The listing builds one solid part. Answer for the finished solid, in the listing's coordinates (mm). Face numbers are marked on the shaded views. Coordinates: 2 decimals unless noted, no trailing zeros. Order: outer loops, then holes, each group sorted by start corner. A loop starts at its lowest first (then second) coordinate and runs counter-clockwise, first axis right, second up. Notation, with made-up numbers: M 52.25,18 L 95.25,18 A22 cw 95.25,29 Z; hole C -34.75,20 d9. An arc over 180 degrees is marked long. One line per item, written item: value. Start each with the question number.
Q1. Determine the mould class of the marked faces 1, 2 and 3 for opening direction X: pulls with the +X half, pulls with the -X half, needs draft (parallel to the pull), parting line crosses it, or undercut.
Q2. The part is cut by section C-C on y = -162. Give the vertices of the cut face in (x, z) (3 decimals).
Q3. Each of these flat-tipped pins is pushed along its axis until it touches: pin 1 Ø11.5 at (x, y) = (-90.4, -156.19) entering from -Z; pin 2 Ø1.5 at (x, z) = (-77.5, 0.5) entering from -Y. Where does it stop, or does it pass through?
Q4. Straight lines are drawn through the part: line 1 along X through (y, z) = (-133.5, 0.65); line 2 along Y through (x, z) = (-100.5, 1.05); line 3 along Y through (x, z) = (-87, 0.25). For each, find the intervals that lie inside material, in ascending order. Write a range as [from, to].
Q5. The part is cut by section A-A on x = -89. Give the vertices of the cut face in (y, z) (3 decimals), then the cut area to 3 significant figures.
Q6. The part is cut by section B-B on z = 2.6. Give the number of separate pieces and of enclosed holes in the cut face, then the cut area to 3 significant figures.
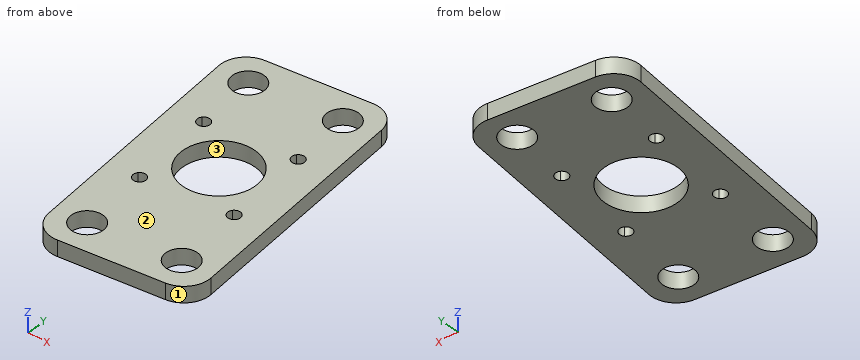
```python
from build123d import *

# Parameters (mm, degrees)
SKETCH1_R           = 7.317167392
SKETCH1_R_2         = 3.175
BOSS_EXTRUDE2_DEPTH = 3.175


with BuildPart() as part:
    # Sketch1 → Boss-Extrude2 (new body)
    with BuildSketch(Plane.XY):
        with BuildLine():
            ThreePointArc((-108.18478159, -135.764097779), (-107.141377815, -132.018654189), (-103.75515137, -130.108023512))
            Line((-103.75515137, -130.108023512), (-83.685324569, -127.667488038))
            ThreePointArc((-83.685324569, -127.667488038), (-79.939880979, -128.710891812), (-78.029250302, -132.097118258))
            Line((-78.029250302, -132.097118258), (-72.356946589, -178.743501511))
            ThreePointArc((-72.356946589, -178.743501511), (-73.400350364, -182.488945101), (-76.78657681, -184.399575778))
            Line((-76.78657681, -184.399575778), (-96.85640361, -186.840111252))
            ThreePointArc((-96.85640361, -186.840111252), (-100.6018472, -185.796707477), (-102.512477877, -182.410481032))
            Line((-102.512477877, -182.410481032), (-108.18478159, -135.764097779))
        make_face()
        with Locations((-90.400440681, -156.188222118)):
            Circle(SKETCH1_R, mode=Mode.SUBTRACT)
        with Locations((-96.362218078, -180.383240442)):
            Circle(SKETCH1_R_2, mode=Mode.SUBTRACT)
        with Locations((-78.813817399, -178.249315979)):
            Circle(SKETCH1_R_2, mode=Mode.SUBTRACT)
        with Locations((-84.179510101, -134.124358848)):
            Circle(SKETCH1_R_2, mode=Mode.SUBTRACT)
        with Locations((-101.72791078, -136.258283311)):
            Circle(SKETCH1_R_2, mode=Mode.SUBTRACT)
        with BuildLine():
            ThreePointArc((-99.257486995, -149.251707821), (-99.470879442, -147.496867753), (-101.225719509, -147.710260199))
            ThreePointArc((-101.225719509, -147.710260199), (-101.012327063, -149.465100267), (-99.257486995, -149.251707821))
        make_face(mode=Mode.SUBTRACT)
        with BuildLine():
            ThreePointArc((-83.677318831, -145.576335736), (-83.463926384, -147.331175804), (-81.709086316, -147.117783358))
            ThreePointArc((-81.709086316, -147.117783358), (-81.922478763, -145.36294329), (-83.677318831, -145.576335736))
        make_face(mode=Mode.SUBTRACT)
        with BuildLine():
            ThreePointArc((-79.575161853, -164.666184037), (-79.7885543, -162.911343969), (-81.543394368, -163.124736415))
            ThreePointArc((-81.543394368, -163.124736415), (-81.330001921, -164.879576483), (-79.575161853, -164.666184037))
        make_face(mode=Mode.SUBTRACT)
        with BuildLine():
            ThreePointArc((-99.091795046, -165.258660878), (-98.8784026, -167.013500946), (-97.123562532, -166.8001085))
            ThreePointArc((-97.123562532, -166.8001085), (-97.336954979, -165.045268432), (-99.091795046, -165.258660878))
        make_face(mode=Mode.SUBTRACT)
    extrude(amount=BOSS_EXTRUDE2_DEPTH)


solid = part.part
```
Output:
1. face 1: pulls with the +X half
1. face 2: needs draft
1. face 3: undercut
2. outline: M -104.994,0 L -94.846,0 L -94.846,3.175 L -104.994,3.175 Z; M -85.955,0 L -74.393,0 L -74.393,3.175 L -85.955,3.175 Z
3. pin 1: passes through
3. pin 2: stops at y = -184.58
4. line 1: x = [-107.95, -103.3], [-100.16, -87.29], [-81.07, -77.86]
4. line 2: y = [-185.87, -149.7], [-147.26, -139.19], [-133.33, -129.71]
4. line 3: y = [-185.64, -162.67], [-149.71, -135.58], [-132.67, -128.07]
5. outline: M -185.885,0 L -163.37,0 L -163.37,3.175 L -185.885,3.175 Z; M -149.006,0 L -128.314,0 L -128.314,3.175 L -149.006,3.175 Z
5. area: 137 mm^2
6. separate pieces: 1
6. enclosed holes: 9
6. area: 1,400 mm^2
